from build123d import *

# Parameters (mm, degrees)
F0_R     = 8.5
F1_DEPTH = 4
F2_R     = 5
F3_DEPTH = 100
F4_W     = 4
F4_H     = 5
F6_W     = 4
F6_H     = 36.891641
F7_DEPTH = 1


with BuildPart() as f1:
    # F0 (on Top) → F1 (new body)
    with BuildSketch(Plane.XY):
        Circle(F0_R)
    extrude(amount=F1_DEPTH)

    # F2 (on Top) → F3 (join)
    with BuildSketch(Plane.XY):
        Circle(F2_R)
    extrude(amount=F3_DEPTH)

    # F4 (on Right) → F5 (revolve)
    with BuildSketch(Plane.YZ):
        with Locations((2, 102.5)):
            Rectangle(F4_W, F4_H)
    revolve(axis=Axis((0, 0, 102.5), (0, 0, -1)))

    # F6 (on face) → F7 (cut)
    with BuildSketch(Plane(origin=(0, 0, 0), x_dir=(1, 0, 0), z_dir=(0, 0, -1))):
        with Locations((6, -0.745802)):
            Rectangle(F6_W, F6_H)
    extrude(amount=-F7_DEPTH, mode=Mode.SUBTRACT)


solid = f1.part
Build history of the part. All positions in model axes, mm. A direction names the side the tool comes from. Round coordinates to 2 decimals unless told otherwise and drop trailing zeros. Loops run counter-clockwise (first coordinate to the right, second up) from the corner with the lowest first, then second, coordinate; pieces in that order, holes last. Notation, with made-up numbers: (55.5, 36) -> (62.5, 36) arc R31 cw to (62.5, 69) -> close; hole circle Ø5 at (89, 28.5). An arc over 180 degrees is marked (long way). Use CSV: the item, a comma, the result in double quotes. Start each with the question number.
Q1. Saw through at C-C on z = 14. Give the cut face in (x, y).
Q2. Mould opens along X. For faces 1 (the face through (4, -4, 4)), 2 (the face through (6, 0, 1)), 3 (the face through (-8.49, 0.37, 1.97)) say: +X half, -X half, draft (parallel to the pull), parting line (faces both ways), or undercut.
Q3. Saw through at D-D on y = -6. Give the cut face in (x, z).
Q4. Flat gauge pins, fed straight in: pin 1 Ø1.2 at (x, y) = (6, -0.5) entering from -Z; pin 2 Ø4 at (y, z) = (-0.5, 60.5) entering from +X; pin 3 Ø1.5 at (x, y) = (6.5, 0.5) entering from +Z; pin 4 Ø2 at (x, y) = (-4, -0.5) entering from -Z. Where does each tip first touch, or does it go through?
Q5. Saw through at A-A on y = 0. Give the cut face in (x, z).
Q6. Which spindle directions (+Z, -Z, +X, -X, +Y, -Y) get a long thin tool onto all of the face, cutting with end or side? Do faces 4 (the face through (-3.905, -0.867, 102.535)), 5 (the face through (0, 0, 105)). Say none if no direction does.
Q7. Drill centre lines: L1, parallel to Z at x = -0.75, y = 6.5; L2, parallel to X at y = 3, z = 28; L3, parallel to Z at x = 4.5, y = -7. Where is each one in solid material? Low to high.
Q8. Saw through at B-B on x = 0. Give the cut face in (y, z), and give its area (3 significant figures).
Solutions:
1,outline,"circle Ø10 at (0, 0)"
2,face 1,"draft"
2,face 2,"undercut"
2,face 3,"parting line"
3,outline,"(-6.02, 0) -> (4, 0) -> (4, 1) -> (6.02, 1) -> (6.02, 4) -> (-6.02, 4) -> close"
4,pin 1,"stops at z = 1"
4,pin 2,"stops at x = 5"
4,pin 3,"stops at z = 4"
4,pin 4,"stops at z = 0"
5,outline,"(-8.5, 0) -> (4, 0) -> (4, 1) -> (8, 1) -> (8, 0) -> (8.5, 0) -> (8.5, 4) -> (5, 4) -> (5, 100) -> (4, 100) -> (4, 105) -> (-4, 105) -> (-4, 100) -> (-5, 100) -> (-5, 4) -> (-8.5, 4) -> close"
6,face 4,"+Z"
6,face 5,"+Z, +X, -X, +Y, -Y"
7,L1,"z = 0 to 4"
7,L2,"x = -4 to 4"
7,L3,"z = 1 to 4"
8,outline,"(-8.5, 0) -> (8.5, 0) -> (8.5, 4) -> (5, 4) -> (5, 100) -> (4, 100) -> (4, 105) -> (-4, 105) -> (-4, 100) -> (-5, 100) -> (-5, 4) -> (-8.5, 4) -> close"
8,area,"1,070 mm^2"
